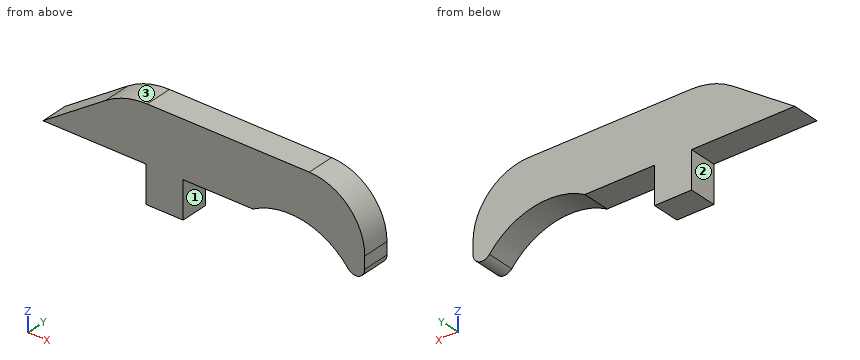
```python
from build123d import *

# Parameters (mm, degrees)
BOSS_EXTRUDE1_DEPTH = 4.7625
FILLET1_R           = 9.525
FILLET2_R           = 1.5875
FILLET4_R           = 12.7
SKETCH2_W           = 6.35
SKETCH2_H           = 6.35
BOSS_EXTRUDE2_DEPTH = 4.7625


with BuildPart() as part:
    # Sketch1 → Boss-Extrude1 (new body)
    with BuildSketch(Plane(origin=(0, 0, 0), x_dir=(1, 0, 0), z_dir=(0, 1, 0))):
        with BuildLine():
            ThreePointArc((58.42, 11.1252), (52.020983, 0.025067), (39.208499, 0))
            Line((39.208499, 0), (3.175, 0))
            Line((3.175, 0), (17.145, -9.525))
            Line((17.145, -9.525), (58.42, -9.525))
            Line((58.42, -9.525), (58.42, 11.1252))
        make_face()
    extrude(amount=BOSS_EXTRUDE1_DEPTH)

    # Fillet1
    fillet1_edges = [part.edges().sort_by_distance(p)[0] for p in [
        (58.42, 2.38125, 9.525),
    ]]
    fillet(fillet1_edges, radius=FILLET1_R)

    # Fillet2
    fillet2_edges = [part.edges().sort_by_distance(p)[0] for p in [
        (58.42, 2.38125, -11.1252),
    ]]
    fillet(fillet2_edges, radius=FILLET2_R)

    # Fillet4
    fillet4_edges = [part.edges().sort_by_distance(p)[0] for p in [
        (17.145, 2.38125, 9.525),
    ]]
    fillet(fillet4_edges, radius=FILLET4_R)

    # Sketch2 → Boss-Extrude2 (add)
    with BuildSketch(Plane.XZ):
        with Locations((24.0645, -3.175)):
            Rectangle(SKETCH2_W, SKETCH2_H)
    extrude(amount=-BOSS_EXTRUDE2_DEPTH)


solid = part.part
```
CAD build for the part. Positions are in the model's coordinates, mm. Face numbers are marked on the shaded views. A direction names the side the tool comes from. Round coordinates to 2 decimals unless told otherwise and drop trailing zeros. Loops run counter-clockwise (first coordinate to the right, second up) from the corner with the lowest first, then second, coordinate; pieces in that order, holes last. Notation, with made-up numbers: (76.5, 34) - (105.5, 34) arc R14 ccw to (105.5, 61) - close; hole circle Ø1 at (76.5, -20). An arc over 180 degrees is marked (long way). Return JSON: item names as keys, results as strings. Group by question number.
Q1. Flat gauge pin, fed straight in: pin 1 Ø2.5 at (y, z) = (3, -4) entering from -X. Where does the tip first touch, or does it go through?
Q2. Band-saw the part on D-D on z = 3. Give the cut face in (x, y) (1 decimal).
Q3. Band-saw the part on C-C on x = 42. Give the cut face in (y, z) (1 decimal).
Q4. Tool access for the marked faces 1, 2 and 3: list every direction of +Z, -Z, +X, -X, +Y, -Y with a clear straight run to the whole face (end or side of a thin tool).
Q5. Band-saw the part on B-B on z = -0.75. Give the cut face in (x, y), plus the area to 3 significant figures.
Q6. Drill centre lines: line 1 along X through (y, z) = (4.45, -4); line 2 along Z through (x, y) = (38, 0.5) (3 decimals); line 3 along X through (y, z) = (2.5, -0.25). Where is each one in solid material? Low to high. Write a range as [from, to].
Solutions:
{
 "1": {"pin 1": "stops at x = 20.89"},
 "2": {"outline": "(7.6, 0) - (57.9, 0) - (57.9, 4.8) - (7.6, 4.8) - close"},
 "3": {"outline": "(0, 1.2) - (4.8, 1.2) - (4.8, 9.5) - (0, 9.5) - close"},
 "4": {"face 1": "-Z, +Y, -Y", "face 2": "-Z, -X, +Y, -Y", "face 3": "+Z, -X, +Y, -Y"},
 "5": {"outline": "(20.89, 0) - (27.24, 0) - (27.24, 4.76) - (20.89, 4.76) - close; (53.14, 0) - (58.42, 0) - (58.42, 4.76) - (53.14, 4.76) - close", "area": "55.4 mm^2"},
 "6": {"line 1": "x = [20.89, 27.24]", "line 2": "z = [0, 9.525]", "line 3": "x = [20.89, 27.24], [52.39, 58.42]"}
}
